from build123d import *

# Parameters (mm, degrees)
SKETCH1_R           = 2.35
SKETCH1_R_2         = 2.3
BOSS_EXTRUDE2_DEPTH = 3
SKETCH2_W           = 4.283202477
SKETCH2_H           = 3
BOSS_EXTRUDE3_DEPTH = 2.5
BOSS_EXTRUDE4_DEPTH = 10.5
FILLET1_R           = 1
SKETCH4_W           = 4.283202477
SKETCH4_H           = 7.5
CUT_EXTRUDE1_DEPTH  = 0.25


with BuildPart() as part:
    # Sketch1 → Boss-Extrude2 (new body)
    with BuildSketch(Plane.XY.offset(-130.24387898)):
        with BuildLine():
            Line((-15.010059364, 38.189351968), (-15.708117617, 37.572463316))
            ThreePointArc((-15.708117617, 37.572463316), (-16.257044738, 28.67984396), (-7.364425381, 28.130916839))
            Line((-7.364425381, 28.130916839), (-4.154897186, 30.967244081))
            ThreePointArc((-4.154897186, 30.967244081), (-3.141509811, 33.204488286), (-4.138848078, 35.44893298))
            ThreePointArc((-4.138848078, 35.44893298), (-9.854378586, 43.268649811), (-11.908958835, 52.734058429))
            ThreePointArc((-11.908958835, 52.734058429), (-12.792945326, 54.845611755), (-14.908920841, 55.718960016))
            Line((-14.908920841, 55.718960016), (-23.716053845, 55.718960016))
            ThreePointArc((-23.716053845, 55.718960016), (-28.216053845, 51.218960016), (-23.716053845, 46.718960016))
            Line((-23.716053845, 46.718960016), (-19.942226175, 46.718960016))
            ThreePointArc((-19.942226175, 46.718960016), (-18.729620599, 46.309427783), (-18.013616093, 45.248547734))
            ThreePointArc((-18.013616093, 45.248547734), (-16.74918621, 41.617962479), (-15.010059364, 38.189351968))
        make_face()
        with Locations((-23.716053845, 51.218960016)):
            Circle(SKETCH1_R, mode=Mode.SUBTRACT)
        with Locations((-11.536271499, 32.851690078)):
            Circle(SKETCH1_R_2, mode=Mode.SUBTRACT)
    extrude(amount=BOSS_EXTRUDE2_DEPTH)

    # Sketch2 → Boss-Extrude3 (add)
    with BuildSketch(Plane(origin=(-17.188019546, 19.449601065, 0), x_dir=(0.7493290854811405, 0.6621977964717171, 0), z_dir=(0.6621977964717171, -0.7493290854811405, 0))):
        with Locations((15.251454246, -128.74387898)):
            Rectangle(SKETCH2_W, SKETCH2_H)
    extrude(amount=BOSS_EXTRUDE3_DEPTH)

    # Sketch3 → Boss-Extrude4 (add)
    with BuildSketch(Plane.XY.offset(-127.24387898)):
        Polygon((-7.364425381, 28.130916839), (-4.154897186, 30.967244081), (-2.499402695, 29.093921367), (-5.70893089, 26.257594125), align=None)
    extrude(amount=-BOSS_EXTRUDE4_DEPTH)

    # Fillet1
    fillet1_edges = [part.edges().sort_by_distance(p)[0] for p in [
        (-5.70893089, 26.257594125, -132.49387898),
        (-2.499402695, 29.093921367, -132.49387898),
    ]]
    fillet(fillet1_edges, radius=FILLET1_R)

    # Sketch4 → Cut-Extrude1 (cut)
    with BuildSketch(Plane(origin=(-17.188019546, 19.449601065, 0), x_dir=(0.7493290854811406, 0.6621977964717171, 0), z_dir=(-0.6621977964717171, 0.7493290854811406, 0))):
        with Locations((15.251454246, 133.99387898)):
            Rectangle(SKETCH4_W, SKETCH4_H)
    extrude(amount=-CUT_EXTRUDE1_DEPTH, mode=Mode.SUBTRACT)


solid = part.part
Design review of the part built by this model. Coordinates are the model's own, in mm. A direction names the side the tool comes from. Give positions to 0.01 mm unless a question says otherwise; leave off trailing zeros. Write each loop counter-clockwise with the first axis right and the second up, starting at its lowest first coordinate (ties: lowest second). Pieces come first, ordered by that corner, then holes. Notation, with made-up numbers: M 68.5,-29.5 L 83.5,-29.5 A30 cw 83.5,-4.5 Z; hole C 89.5,39.25 d9. An arc over 180 degrees is marked long. Return JSON: item names as keys, results as strings. Group by question number.
Item 1: Take a section at D-D (x = -20.75). Give the boundary of the cut face in (y, z), plus the area to 3 significant figures.
Item 2: Tool access review of faces 1 (the cylindrical face through (-16.77, 41.67, -128.76)), 2 (the cylindrical face through (-16.348, 28.785, -128.765)): name each direction out of +Z, -Z, +X, -X, +Y, -Y from which nothing blocks a thin tool from reaching the whole face with its end or side.
Item 3: The part is to be moulded in two halves that separate along Y. For faces 3 (the flat face through (-5.62, 29.34, -134.05)), 4 (the flat face through (-15, 42, -127.244)), 5 (the flat face through (-22, 46.719, -129)), 6 (the cylindrical face through (-3.14, 33.17, -128.76)), say which applies: pulls with the +Y half, pulls with the -Y half, needs draft (parallel to the pull), parting line crosses it, or undercut.
Item 4: Take a section at A-A (x = -10.25). Give the boundary of the cut face in (y, z), plus the area to 3 significant figures.
Item 5: Wall thickness on line 1 along Z through (x, y) = (-14.75, 36.25); line 2 along X through (y, z) = (32, -130); line 3 along X through (y, z) = (47.25, -129.5): over which ranges is each line inside the solid? List them lowest first.
Item 6: Take a section at B-B (y = 34.5). Give the boundary of the cut face in (x, z).
Item 7: Take a section at C-C (z = -133.25). Give the boundary of the cut face in (x, y), plus the area to 3 significant figures.
Item 8: Clearance check with flat-ended pins moving along their axes: pin 1 Ø8 at (x, y) = (-24.5, 47.5) entering from -Z; pin 2 Ø1.5 at (x, z) = (-22.5, -129) entering from -Y; pin 3 Ø3 at (x, z) = (-14.5, -128.5) entering from -Y. State where each tip first meets the part, or that it passes through.
Return value:
{
 "1": {"outline": "M 46.72,-130.24 L 55.72,-130.24 L 55.72,-127.24 L 46.72,-127.24 Z", "area": "27.0 mm2"},
 "2": {"face 1": "+Z, -Z, -X", "face 2": "+Z, -Z"},
 "3": {"face 3": "pulls with the +Y half", "face 4": "needs draft", "face 5": "pulls with the -Y half", "face 6": "undercut"},
 "4": {"outline": "M 26.68,-130.24 L 30.94,-130.24 L 30.94,-127.24 L 26.68,-127.24 Z; M 34.76,-130.24 L 44.2,-130.24 L 44.2,-127.24 L 34.76,-127.24 Z", "area": "41.1 mm2"},
 "5": {"line 1": "z = -130.24 to -127.24", "line 2": "x = -17.78 to -13.67, -9.4 to -3.4", "line 3": "x = -25.84 to -11.23"},
 "6": {"outline": "M -17.62,-130.24 L -13.14,-130.24 L -13.14,-127.24 L -17.62,-127.24 Z; M -9.93,-130.24 L -3.43,-130.24 L -3.43,-127.24 L -9.93,-127.24 Z"},
 "7": {"outline": "M -7.2,27.94 L -6.37,27.01 A1 ccw -4.96,26.92 L -3.25,28.43 A1 ccw -3.16,29.84 L -3.99,30.78 Z", "area": "9.21 mm2"},
 "8": {"pin 1": "stops at z = -130.24", "pin 2": "stops at y = 46.72", "pin 3": "stops at y = 26.72"}
}
